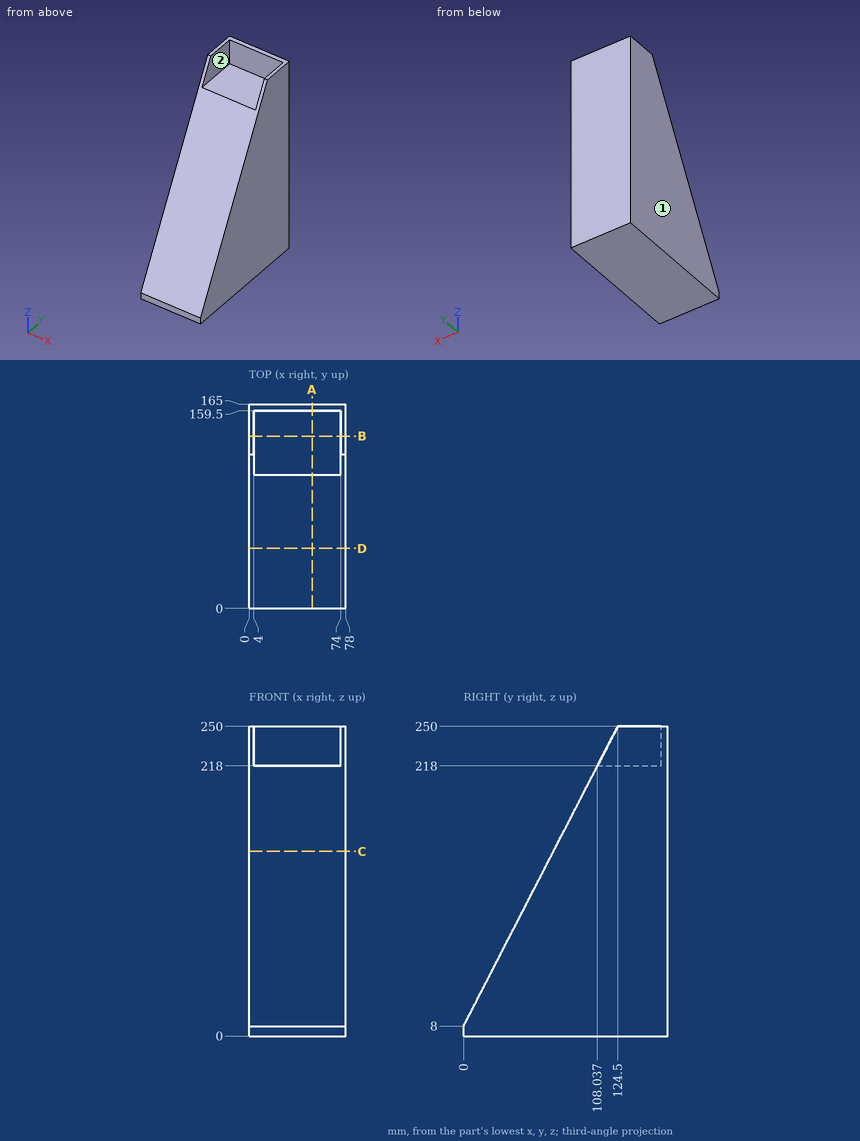
Verification items for this drawing (mm, ordinates from the low corner). A direction names the side the tool comes from. Coordinates: 2 decimals unless noted, no trailing zeros. Order: outer loops, then holes, each group sorted by start corner. A loop starts at its lowest first (then second) coordinate and runs counter-clockwise, first axis right, second up.
Q1. Depth check by flat-ended pin: pin 1 Ø2 at (x, z) = (34, 187.5) entering from -Y; pin 2 Ø4 at (x, y) = (39, 59) entering from +Z; pin 3 Ø5 at (x, z) = (35.5, 186.5) entering from -Y (1 decimal). Enter the tip coordinate at first touch or a pass-through.
Reply:
pin 1: stops at y = 91.83
pin 2: stops at z = 126.57
pin 3: stops at y = 90.5
Q2. Thickness scan on probe 1 along X at (y, z) = (157.5, 225.5); probe 2 along Z at (x, y) = (38.5, 146); probe 3 along Z at (x, y) = (54.5, 58). Record the ranges inside material, lowest first.
Reply:
probe 1: x = 0 to 4, 74 to 78
probe 2: z = 0 to 218
probe 3: z = 0 to 120.74
Q3. Sectioned sample at C-C on z = 149. Record the cut outline in (x, y).
Reply:
outline: (0, 72.54) - (78, 72.54) - (78, 165) - (0, 165) - close
Q4. Sectioned sample at B-B on y = 139. Record the cut outline in (x, z).
Reply:
outline: (0, 0) - (78, 0) - (78, 250) - (74, 250) - (74, 218) - (4, 218) - (4, 250) - (0, 250) - close
Q5. Sectioned sample at A-A on x = 51. Record the cut outline in (y, z).
Reply:
outline: (0, 0) - (165, 0) - (165, 250) - (159.5, 250) - (159.5, 218) - (108.04, 218) - (0, 8) - close
Q6. Sectioned sample at D-D on y = 48.5. Record the cut outline in (x, z), and give its area (3 significant figures).
Reply:
outline: (0, 0) - (78, 0) - (78, 102.27) - (0, 102.27) - close
area: 7,980 mm2
Q7. Tool access check on the marked faces 1 and 2. Record the directions out of +Z, -Z, +X, -X, +Y, -Y that give a thin tool (end or side, any length) a straight path to the whole face; none if there is none.
Reply:
face 1: +Z, -Z, -X, +Y, -Y
face 2: +Z, -Y
